Geometry check sheet. Reference: drawing and pictorial views, mm from the part's lowest x, y, z. Round coordinates to 2 decimals unless told otherwise and drop trailing zeros. Order: outer loops, then holes, each group sorted by start corner. A loop starts at its lowest first (then second) coordinate and runs counter-clockwise, first axis right, second up.
Q1. Cross-section at D-D on y = 104. Record the cut outline in (x, z).
Q2. Cross-section at B-B on y = 41. Record the cut outline in (x, z).
Q3. Cross-section at A-A on x = 79.5. Record the cut outline in (y, z), then the cut area to 3 significant figures.
Q4. Cross-section at C-C on z = 5.5. Record the cut outline in (x, y).
Q5. Depth check by flat-ended pin: P1, Ø4.5, axis at y = 102, z = 1, coming from the -X side; P2, Ø2.5, axis at x = 91, y = 93.5, coming from the -Z side. Enter the tip coordinate at first touch or a pass-through.
Q6. Scan lines: probe 1 along X at (y, z) = (10.5, 5.75); probe 2 along Y at (x, z) = (73, 3.75); probe 3 along X at (y, z) = (47.5, 1.5). Record each from-to range of solid material in increasing order.
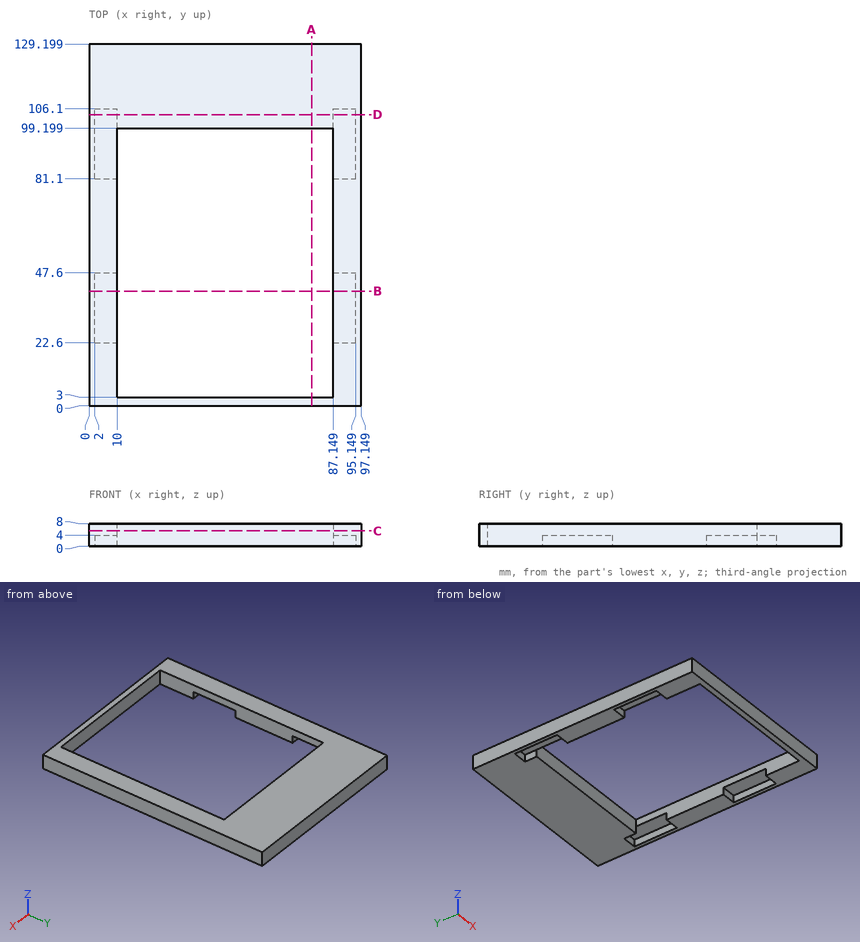
Results found:
1. outline: (0, 0) - (2, 0) - (2, 4) - (10, 4) - (10, 0) - (87.15, 0) - (87.15, 4) - (95.15, 4) - (95.15, 0) - (97.15, 0) - (97.15, 8) - (0, 8) - close
2. outline: (0, 0) - (2, 0) - (2, 4) - (10, 4) - (10, 8) - (0, 8) - close; (87.15, 4) - (95.15, 4) - (95.15, 0) - (97.15, 0) - (97.15, 8) - (87.15, 8) - close
3. outline: (0, 0) - (3, 0) - (3, 8) - (0, 8) - close; (99.2, 0) - (129.2, 0) - (129.2, 8) - (99.2, 8) - close
3. area: 264 mm2
4. outline: (0, 0) - (97.15, 0) - (97.15, 129.2) - (0, 129.2) - close; hole (10, 3) - (87.15, 3) - (87.15, 99.2) - (10, 99.2) - close
5. P1: stops at x = 0
5. P2: stops at z = 4
6. probe 1: x = 0 to 10, 87.15 to 97.15
6. probe 2: y = 0 to 3, 99.2 to 129.2
6. probe 3: x = 0 to 2, 95.15 to 97.15
